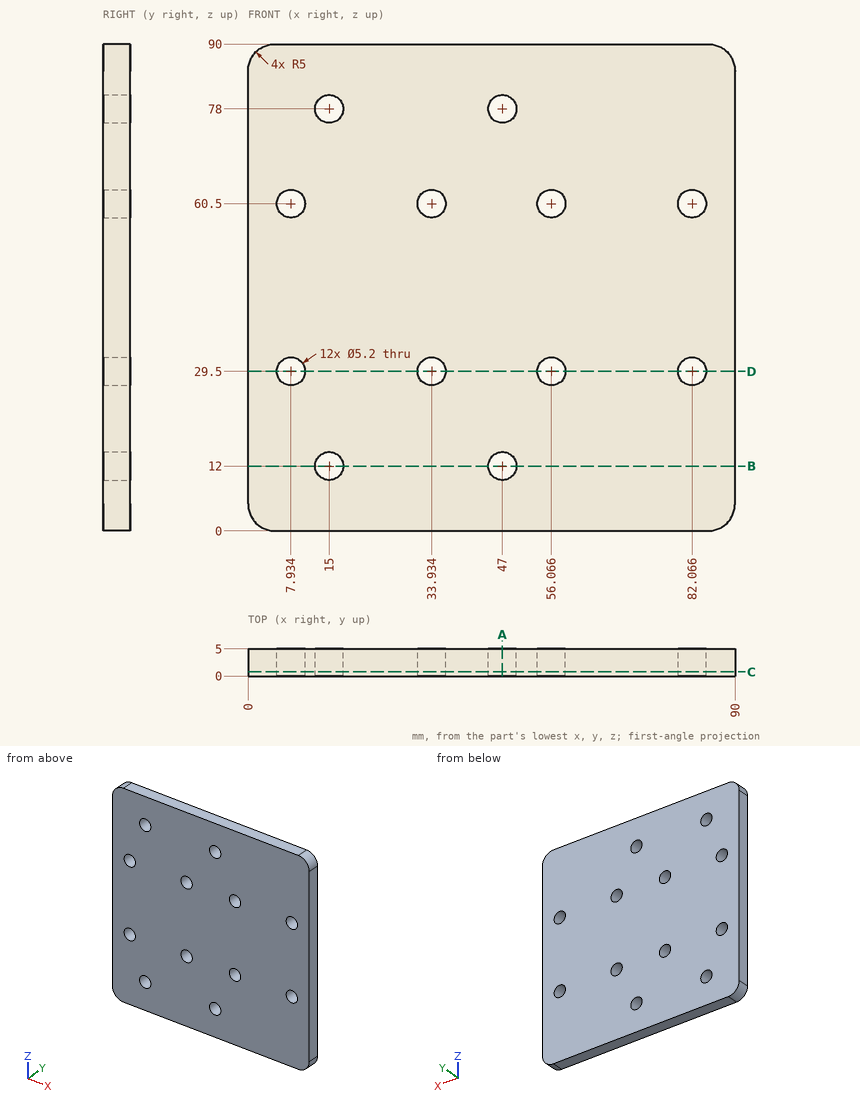
Print and shaded views of the part. All mm, measured from the part's lowest x, y and z. Round coordinates to 2 decimals unless told otherwise and drop trailing zeros. Loops run counter-clockwise (first coordinate to the right, second up) from the corner with the lowest first, then second, coordinate; pieces in that order, holes last. Notation, with made-up numbers: M 27.5,-8 L 65.5,-8 A27 ccw 65.5,22 Z; hole C -20,25 d7. An arc over 180 degrees is marked long. One line per question, with ' | ' between items.
1) Flat gauge pins, fed straight in: pin 1 (4.5 mm diameter, centred on x = 33.93, z = 29.5, fed in from -Y); pin 2 (7 mm diameter, centred on x = 56.07, z = 29.5, fed in from +Y). Where does each tip first touch, or does it go through?
Solved:
pin 1: passes through | pin 2: stops at y = 5
2) Band-saw the part on D-D (z = 29.5). Give the cut face in (x, y).
Solved:
outline: M 0,0 L 5.33,0 L 5.33,5 L 0,5 Z; M 10.53,0 L 31.33,0 L 31.33,5 L 10.53,5 Z; M 36.53,0 L 53.47,0 L 53.47,5 L 36.53,5 Z; M 58.67,0 L 79.47,0 L 79.47,5 L 58.67,5 Z; M 84.67,0 L 90,0 L 90,5 L 84.67,5 Z
3) Band-saw the part on A-A (x = 47). Give the cut face in (y, z), then the cut area to 3 significant figures.
Solved:
outline: M 0,0 L 5,0 L 5,9.4 L 0,9.4 Z; M 0,14.6 L 5,14.6 L 5,75.4 L 0,75.4 Z; M 0,80.6 L 5,80.6 L 5,90 L 0,90 Z | area: 398 mm²
4) Drill centre lines: line 1 along Z through (x, y) = (15, 3); line 2 along Z through (x, y) = (46, 2.75); line 3 along X through (y, z) = (2.3, 58.5) (1 decimal). Where is each one in solid material? Low to high.
Solved:
line 1: z = 0 to 9.4, 14.6 to 75.4, 80.6 to 90 | line 2: z = 0 to 9.6, 14.4 to 75.6, 80.4 to 90 | line 3: x = 0 to 6.3, 9.6 to 32.3, 35.6 to 54.4, 57.7 to 80.4, 83.7 to 90
5) Band-saw the part on C-C (y = 0.75). Give the number of separate pieces and of enclosed holes in the cut face, then the cut area to 3 significant figures.
Solved:
separate pieces: 1 | enclosed holes: 12 | area: 7,820 mm²
6) Band-saw the part on B-B (z = 12). Give the cut face in (x, y).
Solved:
outline: M 0,0 L 12.4,0 L 12.4,5 L 0,5 Z; M 17.6,0 L 44.4,0 L 44.4,5 L 17.6,5 Z; M 49.6,0 L 90,0 L 90,5 L 49.6,5 Z
